Work out the finished part from the listing and answer in its coordinate system (mm). A direction names the side the tool comes from. Round coordinates to 2 decimals unless told otherwise and drop trailing zeros. Loops run counter-clockwise (first coordinate to the right, second up) from the corner with the lowest first, then second, coordinate; pieces in that order, holes last. Notation, with made-up numbers: (14, -9.75) - (52, -9.75) arc R21 cw to (52, 14.25) - close; hole circle Ø10 at (88, 11). An arc over 180 degrees is marked (long way). Return JSON: item names as keys, results as strings.
Autodesk Inventor part; units mm, degrees
ref_plane "Work Plane1" through (0, 0, 25) normal (0, 0, -1) x (-1, 0, 0)
ref_plane "YZ Plane" through (0, 0, 0) normal (1, 0, 0) x (0, 1, 0)
ref_plane "XZ Plane" through (0, 0, 0) normal (0, 1, 0) x (-1, 0, 0)
sketch "Sketch1" plane through (0, 0, 0) normal (0, 1, 0) x (-1, 0, 0)
  line L0 (0, 0) -> (-3, 0)
  line L1 (-3, 0) -> (-3, 50)
  line L2 (-3, 50) -> (0, 50)
  line L3 (0, 50) -> (0, 0)
  dimension "d0" = 50
  dimension "d1" = 6
revolve "Revolution1" add sketch "Sketch1" angle 360 about axis through (0, 0, 50) along (0, 0, -1)
sketch "Sketch2" plane through (0, 0, 0) normal (0, 0, -1) x (-1, 0, 0)
  point P0 (0, 0)
  point P1 (0, 0)
hole "Hole1" at (0, 0, 0) direction (0, 0, 1) diameter 2.459 depth 6 tip angle 118 countersink diameter 4 countersink angle 90
ref_plane "Work Plane1" through (0, 0, 25) normal (0, 0, -1) x (-1, 0, 0)
mirror "Mirror1" about plane through (0, 0, 25) normal (0, 0, -1) of "Hole1"
properties part number "AR-350B" material "Acetal Resin, Black"
1) Section A-A (z = 8) is taken. Give the vertices of the cut face in (x, y), and give its area (3 significant figures).
Verdict:
{"outline": "circle Ø6 at (0, 0)", "area": "28.3 mm2"}
2) Find the intervals of material crossed by L1, parallel to Y at x = 0, z = 48.1; L2, parallel to X at y = -1.75, z = 39, in increasing order.
Verdict:
{"L1": "y = -3 to -1.23, 1.23 to 3", "L2": "x = -2.44 to 2.44"}
3) A tool of negligible diameter and unlimited length cuts with its end or side. For faces 1 (the cylindrical face through (-0.748, -0.976, 46.578)), 2 (the flat face through (1, 2, 50)), from which of +Z, -Z, +X, -X, +Y, -Y can it reach the whole face along a straight path? Write none if from no direction.
Verdict:
{"face 1": "+Z", "face 2": "+Z, +X, -X, +Y, -Y"}
4) Determine the mould class of faces 3 (the cylindrical face through (-3, 0, 25)), 4 (the cylindrical face through (0.748, -0.976, 3.422)), 5 (the flat face through (1, 2, 0)) for opening direction X: pulls with the +X half, pulls with the -X half, needs draft (parallel to the pull), parting line crosses it, or undercut.
Verdict:
{"face 3": "parting line crosses it", "face 4": "undercut", "face 5": "needs draft"}
5) Flat-ended cylindrical pins translate along their axes: pin 1 (1.5 mm diameter, centred on x = -1.5, y = 2, fed in from -Z); pin 2 (1 mm diameter, centred on x = -1.5, z = 6, fed in from -Y); pin 3 (2 mm diameter, centred on y = 1.5, z = 39.5, fed in from -X); pin 4 (2 mm diameter, centred on x = 0, y = 0, fed in from -Z). Find the tip coordinate at first contact, or state that the pin passes through.
Verdict:
{"pin 1": "stops at z = 0", "pin 2": "stops at y = -2.83", "pin 3": "stops at x = -2.96", "pin 4": "stops at z = 6.14"}
